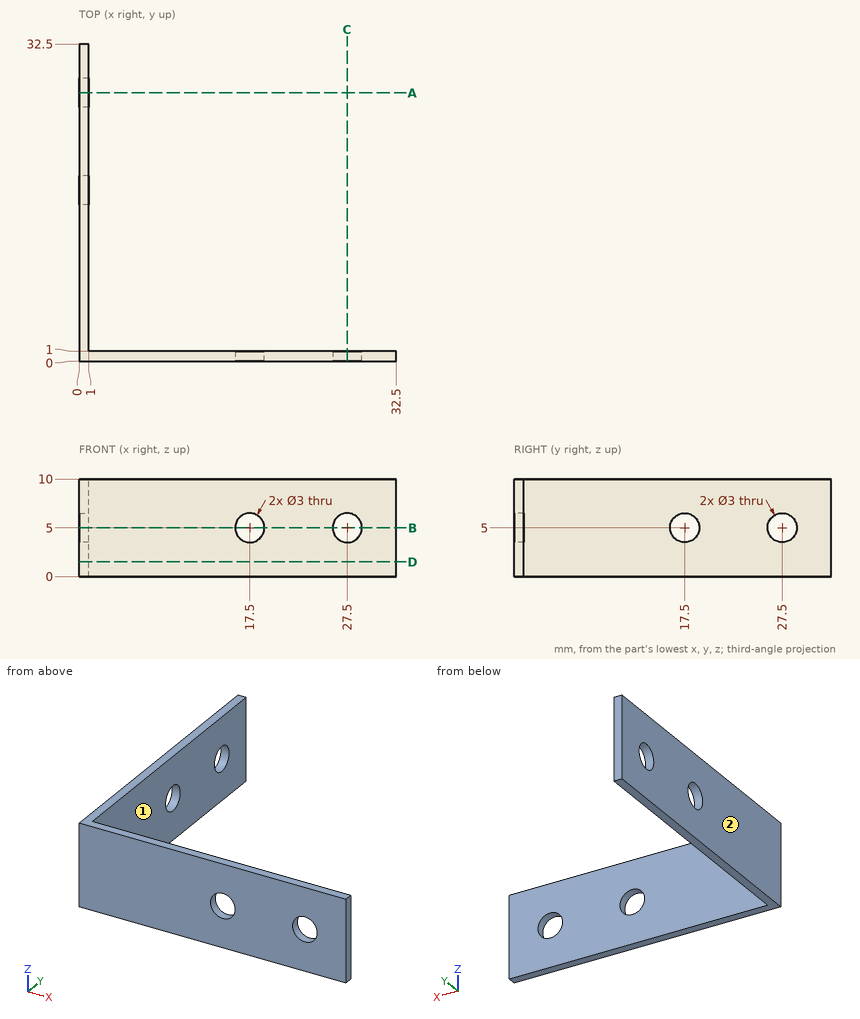
Study the drawing (mm; zero at the part's minimum x, y, z) and answer. A direction names the side the tool comes from. Coordinates: 2 decimals unless noted, no trailing zeros. Order: outer loops, then holes, each group sorted by start corner. A loop starts at its lowest first (then second) coordinate and runs counter-clockwise, first axis right, second up. Notation, with made-up numbers: M 61,-25 L 73,-25 A20 cw 73,2 Z; hole C 78.25,77.25 d4. An arc over 180 degrees is marked long. Answer as a JSON object with one key per item and string values. Group by question number.
1. Section A-A on y = 27.5 is taken. Write down the section's boundary in (x, z).
2. Section D-D on z = 1.5 is taken. Write down the section's boundary in (x, y).
3. Flat-ended cylindrical pins translate along their axes: P1, Ø3, axis at x = 18, z = 3.5, coming from the +Y side; P2, Ø4, axis at y = 9.5, z = 6.5, coming from the +X side. Find the tip coordinate at first contact, or state that the pin passes through.
4. Section B-B on z = 5 is taken. Write down the section's boundary in (x, y), then the cut area to 3 significant figures.
5. A tool of negligible diameter and unlimited length cuts with its end or side. For the marked faces 1 and 2, from which of +Z, -Z, +X, -X, +Y, -Y can it reach the whole face along a straight path? Write none if from no direction.
6. Straight lines are drawn through the part: line 1 (Y direction, x = 0.3, z = 5); line 2 (Z direction, x = 17.5, y = 0.45); line 3 (X direction, y = 15, z = 6). For each, find the intervals that lie inside material, in ascending order.
Values follow:
{
 "1": {"outline": "M 0,0 L 1,0 L 1,3.5 L 0,3.5 Z; M 0,6.5 L 1,6.5 L 1,10 L 0,10 Z"},
 "2": {"outline": "M 0,0 L 32.5,0 L 32.5,1 L 1,1 L 1,32.5 L 0,32.5 Z"},
 "3": {"P1": "y = 1", "P2": "x = 1"},
 "4": {"outline": "M 0,0 L 16,0 L 16,1 L 1,1 L 1,16 L 0,16 Z; M 0,19 L 1,19 L 1,26 L 0,26 Z; M 0,29 L 1,29 L 1,32.5 L 0,32.5 Z; M 19,0 L 26,0 L 26,1 L 19,1 Z; M 29,0 L 32.5,0 L 32.5,1 L 29,1 Z", "area": "52.0 mm2"},
 "5": {"face 1": "+Z, -Z, +X, +Y", "face 2": "+Z, -Z, -X, +Y, -Y"},
 "6": {"line 1": "0 to 16, 19 to 26, 29 to 32.5", "line 2": "0 to 3.5, 6.5 to 10", "line 3": "0 to 1"}
}
